CAD build for the part. Positions are in the model's coordinates, mm. Round coordinates to 2 decimals unless told otherwise and drop trailing zeros. Order: outer loops, then holes, each group sorted by start corner. A loop starts at its lowest first (then second) coordinate and runs counter-clockwise, first axis right, second up. Notation, with made-up numbers: (45, -13) - (70, -13) arc R11 ccw to (70, 5) - close; hole circle Ø9 at (46.5, 41.5). An arc over 180 degrees is marked (long way). Write item = value, one per line.
from build123d import *

# Parameters (mm, degrees)
SKETCH1_W               = 172
SKETCH1_H               = 15
BOSS_EXTRUDE1_DEPTH     = 7.25
CUT_EXTRUDE1_START      = -7.25
SKETCH1_6_W             = 172
SKETCH1_6_H             = 11
CUT_EXTRUDE1_DEPTH      = 3.5
SKETCH2_R               = 1.7
SKETCH2_R_2             = 3
CUT_EXTRUDE2_DEPTH      = 1
CUT_EXTRUDE2_DEPTH_BACK = 8.25
CHAMFER1_SIZE           = 0.4


with BuildPart() as part:
    # Sketch1 → Boss-Extrude1 (new body)
    with BuildSketch(Plane.XY):
        Rectangle(SKETCH1_W, SKETCH1_H)
    extrude(amount=-BOSS_EXTRUDE1_DEPTH)

    # Sketch1<6> → Cut-Extrude1 (cut)
    with BuildSketch(Plane.XY.offset(CUT_EXTRUDE1_START)):
        with Locations((0, -2)):
            Rectangle(SKETCH1_6_W, SKETCH1_6_H)
    extrude(amount=CUT_EXTRUDE1_DEPTH, mode=Mode.SUBTRACT)

    # Sketch2 → Cut-Extrude2 (cut, two sides)
    with BuildSketch(Plane.XY) as cut_extrude2_sk:
        with Locations((-43, 0)):
            Circle(SKETCH2_R)
        Circle(SKETCH2_R)
        with Locations((43, 0)):
            Circle(SKETCH2_R)
        with Locations((-79, 0)):
            Circle(SKETCH2_R_2)
        with Locations((79, 0)):
            Circle(SKETCH2_R_2)
        with Locations((-28, 0)):
            Circle(SKETCH2_R_2)
        with Locations((28, 0)):
            Circle(SKETCH2_R_2)
    extrude(amount=CUT_EXTRUDE2_DEPTH, mode=Mode.SUBTRACT)
    extrude(cut_extrude2_sk.sketch, amount=-CUT_EXTRUDE2_DEPTH_BACK, mode=Mode.SUBTRACT)

    # Chamfer1
    chamfer1_edges = [part.edges().sort_by_distance(p)[0] for p in [
        (76, 0, 0),
        (-82, 0, 0),
        (41.3, 0, 0),
        (-44.7, 0, 0),
        (-31, 0, 0),
        (25, 0, 0),
        (-1.7, 0, 0),
        (0, -7.5, 0),
        (-86, 0, 0),
        (0, 7.5, 0),
        (86, 0, 0),
    ]]
    chamfer(chamfer1_edges, length=CHAMFER1_SIZE)


solid = part.part
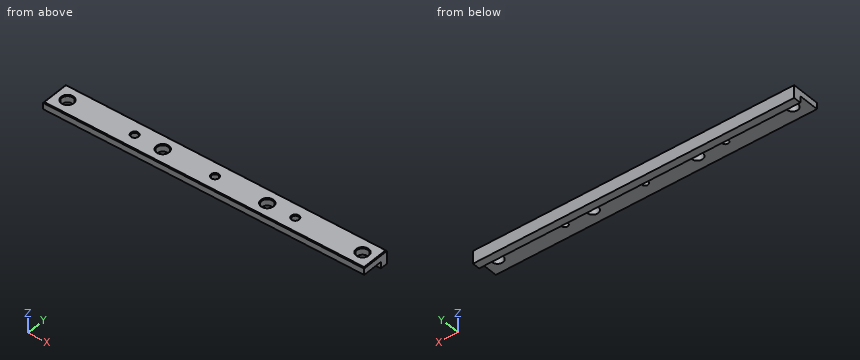
(1) Band-saw the part on C-C on y = 0. Count the separate pieces of the cut face and the enclosed holes in it, plus the area to 3 significant figures.
Solved:
separate_pieces = 8
enclosed_holes = 0
area = 515 mm²
(2) Band-saw the part on D-D on x = 43. List the corners of the cut face in (y, z).
Solved:
outline = (-7.5, -3.75) - (-1.7, -3.75) - (-1.7, -0.4) - (-2.1, 0) - (-7.1, 0) - (-7.5, -0.4) - close; (1.7, -3.75) - (3.5, -3.75) - (3.5, -7.25) - (7.5, -7.25) - (7.5, -0.4) - (7.1, 0) - (2.1, 0) - (1.7, -0.4) - close
(3) Band-saw the part on A-A on x = 79. List the corners of the cut face in (y, z), plus the area to 3 significant figures.
Solved:
outline = (-7.5, -3.75) - (-3, -3.75) - (-3, -0.4) - (-3.4, 0) - (-7.1, 0) - (-7.5, -0.4) - close; (3, -3.75) - (3.5, -3.75) - (3.5, -7.25) - (7.5, -7.25) - (7.5, -0.4) - (7.1, 0) - (3.4, 0) - (3, -0.4) - close
area = 47.4 mm²
(4) Probe line 1 along Y through (x, z) = (-43, -2.7); line 2 along Y through (x, z) = (-79, -2.4); line 3 along Z through (x, y) = (-40.5, -0.5). List the from-to ranges inside material, lowest first.
Solved:
line_1 = -7.5 to -1.7, 1.7 to 7.5
line_2 = -7.5 to -3, 3 to 7.5
line_3 = -3.75 to 0
(5) Band-saw the part on B-B on x = 19.5. List the corners of the cut face in (y, z).
Solved:
outline = (-7.5, -3.75) - (3.5, -3.75) - (3.5, -7.25) - (7.5, -7.25) - (7.5, -0.4) - (7.1, 0) - (-7.1, 0) - (-7.5, -0.4) - close
(6) Drop flat-ended pins along their axis: pin 1 (4.5 mm diameter, centred on x = 0, y = 0, fed in from -Z); pin 2 (1 mm diameter, centred on y = 1, z = -4, fed in from +X). Give the stop position or say it passes through.
Solved:
pin_1 = -3.75
pin_2 = 86
